For this review, take the finished solid that the model builds, in its own axes (mm). Coordinates: 2 decimals unless noted, no trailing zeros. Order: outer loops, then holes, each group sorted by start corner. A loop starts at its lowest first (then second) coordinate and runs counter-clockwise, first axis right, second up. Notation, with made-up numbers: (6.25, 65.5) -> (48.25, 65.5) arc R10 ccw to (48.25, 78.5) -> close; hole circle Ø1 at (17, 63.5). An arc over 180 degrees is marked (long way). Write item = value, one per line. Start each with the question number.
1) Draft analysis for pull direction X (two halves, no side actions). For faces 1 (the face through (-26, 0, -28)), 2 (the face through (-23.122, 295.8, -30.156)), 3 (the face through (-39.05, 295.8, -8.67)), state which applies: +X half, -X half, draft (parallel to the pull), parting line (faces both ways), or undercut.
2) Consider section A-A on x = -26.5. Give the boundary of the cut face in (y, z), and give its area (3 significant figures).
3) Consider section B-B on z = 11.5. Give the boundary of the cut face in (x, y), and give its area (3 significant figures).
4) Insertion check: pin 1 Ø8 at (x, y) = (-5.5, 264.5) entering from +Z; pin 2 Ø4 at (x, y) = (-16, 427.5) entering from +Z; pin 3 Ø6 at (y, z) = (285.5, -26.5) entering from +X. Each pin has a flat end and moves straight along its axis. Give the tip position at first contact, or say it passes through.
5) Consider section C-C on y = 553. Give the boundary of the cut face in (x, z), and give its area (3 significant figures).
6) Wall thickness on probe 1 along X at (y, z) = (464, 0); probe 2 along X at (y, z) = (423, -2.5): over which ranges is each line inside the solid? List them lowest first. Write a range as [from, to].
from build123d import *

# Parameters (mm, degrees)
SKETCH1_R           = 40
SKETCH1_R_2         = 38
BOSS_EXTRUDE1_DEPTH = 600
SKETCH2_W           = 3
SKETCH2_H           = 160
CUT_EXTRUDE1_DEPTH  = 603.660766933
CIRPATTERN1_COUNT   = 4


with BuildPart() as part:
    # Sketch1 → Boss-Extrude1 (new body)
    with BuildSketch(Plane(origin=(0, 0, 0), x_dir=(1, 0, 0), z_dir=(0, 1, 0))):
        with Locations(Location((0, 0, 0), (0, 0, 270))):
            Circle(SKETCH1_R)
        with Locations(Location((0, 0, 0), (0, 0, 270))):
            Circle(SKETCH1_R_2, mode=Mode.SUBTRACT)
    extrude(amount=BOSS_EXTRUDE1_DEPTH)

    # Sketch2 → Cut-Extrude1 (cut, through all)
    with BuildSketch(Plane(origin=(0, 0, 0), x_dir=(0, 0, -1), z_dir=(1, 0, 0))):
        with Locations((0, 80)):
            Rectangle(SKETCH2_W, SKETCH2_H)
    cut_extrude1 = extrude(amount=-CUT_EXTRUDE1_DEPTH, mode=Mode.SUBTRACT)

    # CirPattern1: Cut-Extrude1 ×4 about axis
    cirpattern1_axis = Axis((0, 0, 0), (0, 1, 0))
    for i in range(1, CIRPATTERN1_COUNT):
        add(cut_extrude1.rotate(cirpattern1_axis, i * 360 / CIRPATTERN1_COUNT), mode=Mode.SUBTRACT)


solid = part.part
Answer sheet:
q1.face_1 = draft
q1.face_2 = undercut
q1.face_3 = parting line
q2.outline = (0, -29.96) -> (600, -29.96) -> (600, -27.24) -> (0, -27.24) -> close; (0, 27.24) -> (600, 27.24) -> (600, 29.96) -> (0, 29.96) -> close
q2.area = 3,270 mm2
q3.outline = (-38.31, 0) -> (-36.22, 0) -> (-36.22, 600) -> (-38.31, 600) -> close; (36.22, 0) -> (38.31, 0) -> (38.31, 600) -> (36.22, 600) -> close
q3.area = 2,510 mm2
q4.pin_1 = 39.97
q4.pin_2 = 37.47
q4.pin_3 = 32.37
q5.outline = circle Ø80 at (0, 0); hole circle Ø76 at (0, 0)
q5.area = 490 mm2
q6.probe_1 = [-40, -38], [38, 40]
q6.probe_2 = [-39.92, -37.92], [37.92, 39.92]
